from build123d import *

# Parameters (mm, degrees)
SKETCH1_R               = 55
SKETCH1_W               = 30.631456328
SKETCH1_H               = 90
HOUSING_DEPTH           = 30
INTERNALCUT_DEPTH       = 27
SKETCH7_W               = 72
SKETCH7_H               = 25
DISPLAYCUT_DEPTH        = 27
SKETCH11_R              = 18
WICHARGERCUT_DEPTH      = 1
SKETCH14_W              = 4.6
SKETCH14_H              = 6.1
BTNINTERNALCUT_DEPTH    = 1
SKETCH16_R              = 1.5
BTNEXTERNALCUT_DEPTH    = 116.280995765
SKETCH18_R              = 6
BUZZEREXTERNALCUT_DEPTH = 1
SKETCH20_R              = 0.35
BUZZERINTERNALCUT_DEPTH = 116.863890151
SKETCH23_W              = 3.7
SKETCH23_H              = 8.5
SWITCHINTERNALCUT_DEPTH = 1
SKETCH25_W              = 1.7
SKETCH25_H              = 3.6
SWITCHEXTERNALCUT_DEPTH = 124.821406818
MICROUSBCUT_DEPTH       = 128.13897565
SKETCH29_R              = 3.5
SKETCH29_R_2            = 1.5
BOSS_EXTRUDE1_DEPTH     = 27
SKETCH30_R              = 1.5
CUT_EXTRUDE1_DEPTH      = 83.757833161
CUT_EXTRUDE1_DEPTH_BACK = 83.757833161
SKETCH31_W              = 59.5
SKETCH31_H              = 2
BOSS_EXTRUDE3_DEPTH     = 5


with BuildPart() as part:
    # Sketch1 → Housing (new body)
    with BuildSketch(Plane(origin=(0, 0, 0), x_dir=(1, 0, 0), z_dir=(0, 1, 0))):
        Circle(SKETCH1_R)
        with Locations((40.315728164, -0.0001724)):
            Rectangle(SKETCH1_W, SKETCH1_H)
    extrude(amount=HOUSING_DEPTH)

    # Sketch8 → InternalCut (cut)
    with BuildSketch(Plane(origin=(0, 30, 0), x_dir=(1, 0, 0), z_dir=(0, 1, 0))):
        with BuildLine():
            ThreePointArc((29.731697916, 40.1998276), (-49.999999999, 0.000289929), (29.73123171, -40.2001724))
            Line((29.73123171, -40.2001724), (19.336952431, -40.2001724))
            Line((19.336952431, -40.2001724), (19.336952431, 40.1998276))
            Line((19.336952431, 40.1998276), (29.731697916, 40.1998276))
        make_face()
        with BuildLine():
            Line((19.336952431, -40.2001724), (29.73123171, -40.2001724))
            ThreePointArc((29.73123171, -40.2001724), (44.646173327, -22.510424413), (50, 0))
            ThreePointArc((50, 0), (44.646303855, 22.510165528), (29.731697916, 40.1998276))
            Line((29.731697916, 40.1998276), (19.336952431, 40.1998276))
            Line((19.336952431, 40.1998276), (19.336952431, -40.2001724))
        make_face()
        with BuildLine():
            Line((29.73123171, -40.2001724), (50.631456328, -40.2001724))
            Line((50.631456328, -40.2001724), (50.631456328, 40.1998276))
            Line((50.631456328, 40.1998276), (29.731697916, 40.1998276))
            ThreePointArc((29.731697916, 40.1998276), (44.646303855, 22.510165528), (50, 0))
            ThreePointArc((50, 0), (44.646173327, -22.510424413), (29.73123171, -40.2001724))
        make_face()
    extrude(amount=-INTERNALCUT_DEPTH, mode=Mode.SUBTRACT)

    # Sketch7 → DisplayCut (cut)
    with BuildSketch(Plane(origin=(55.631456328, 0, 0), x_dir=(0, 0, -1), z_dir=(1, 0, 0))):
        with Locations((-0.0001724, 22.5)):
            Rectangle(SKETCH7_W, SKETCH7_H)
    extrude(amount=-DISPLAYCUT_DEPTH, mode=Mode.SUBTRACT)

    # Sketch11 → WiChargerCut (cut)
    with BuildSketch(Plane(origin=(0, 3, 0), x_dir=(1, 0, 0), z_dir=(0, 1, 0))):
        with Locations(Location((0, 0, 0), (0, 0, 270))):
            Circle(SKETCH11_R)
    extrude(amount=-WICHARGERCUT_DEPTH, mode=Mode.SUBTRACT)

    # Sketch14 → BtnInternalCut (cut)
    with BuildSketch(Plane(origin=(4.856972308, 3, -39.46084295), x_dir=(1, 0, 0), z_dir=(0, 1, 0))):
        with Locations((-0.204569722, -74.22253241)):
            Rectangle(SKETCH14_W, SKETCH14_H)
    extrude(amount=-BTNINTERNALCUT_DEPTH, mode=Mode.SUBTRACT)

    # Sketch16 → BtnExternalCut (cut, through all)
    with BuildSketch(Plane(origin=(4.856972308, 2, -39.46084295), x_dir=(1, 0, 0), z_dir=(0, 1, 0))):
        with Locations(Location((-0.204569722, -74.22253241, 0), (0, 0, 270))):
            Circle(SKETCH16_R)
    extrude(amount=-BTNEXTERNALCUT_DEPTH, mode=Mode.SUBTRACT)

    # Sketch18 → BuzzerExternalCut (cut)
    with BuildSketch(Plane(origin=(12.790381818, 3, 34.693395374), x_dir=(1, 0, 0), z_dir=(0, 1, 0))):
        with Locations(Location((-25.006618322, 0, 0), (0, 0, 270))):
            Circle(SKETCH18_R)
    extrude(amount=-BUZZEREXTERNALCUT_DEPTH, mode=Mode.SUBTRACT)

    # Sketch20 → BuzzerInternalCut (cut, through all)
    with BuildSketch(Plane(origin=(12.790381818, 2, 34.693395374), x_dir=(1, 0, 0), z_dir=(0, 1, 0))):
        with Locations(Location((-24.042348329, 4.522315504, 0), (0, 0, 270))):
            Circle(SKETCH20_R)
        with Locations(Location((-26.042348329, 3.020429056, 0), (0, 0, 270))):
            Circle(SKETCH20_R)
        with Locations(Location((-28.042348329, 3.020429056, 0), (0, 0, 270))):
            Circle(SKETCH20_R)
        with Locations(Location((-30.042348329, 1.518542609, 0), (0, 0, 270))):
            Circle(SKETCH20_R)
        with Locations(Location((-30.042348329, 0.016656161, 0), (0, 0, 270))):
            Circle(SKETCH20_R)
        with Locations(Location((-30.042348329, -1.485230286, 0), (0, 0, 270))):
            Circle(SKETCH20_R)
        with Locations(Location((-28.042348329, 0.016656161, 0), (0, 0, 270))):
            Circle(SKETCH20_R)
        with Locations(Location((-28.042348329, 1.518542609, 0), (0, 0, 270))):
            Circle(SKETCH20_R)
        with Locations(Location((-28.042348329, -1.485230286, 0), (0, 0, 270))):
            Circle(SKETCH20_R)
        with Locations(Location((-28.042348329, -2.987116733, 0), (0, 0, 270))):
            Circle(SKETCH20_R)
        with Locations(Location((-26.042348329, 0.016656161, 0), (0, 0, 270))):
            Circle(SKETCH20_R)
        with Locations(Location((-26.042348329, 1.518542609, 0), (0, 0, 270))):
            Circle(SKETCH20_R)
        with Locations(Location((-26.042348329, -1.485230286, 0), (0, 0, 270))):
            Circle(SKETCH20_R)
        with Locations(Location((-26.042348329, -2.987116733, 0), (0, 0, 270))):
            Circle(SKETCH20_R)
        with Locations(Location((-26.042348329, -4.489003181, 0), (0, 0, 270))):
            Circle(SKETCH20_R)
        with Locations(Location((-24.042348329, -4.489003181, 0), (0, 0, 270))):
            Circle(SKETCH20_R)
        with Locations(Location((-24.042348329, -2.987116733, 0), (0, 0, 270))):
            Circle(SKETCH20_R)
        with Locations(Location((-24.042348329, -1.485230286, 0), (0, 0, 270))):
            Circle(SKETCH20_R)
        with Locations(Location((-24.042348329, 0.016656161, 0), (0, 0, 270))):
            Circle(SKETCH20_R)
        with Locations(Location((-24.042348329, 1.518542609, 0), (0, 0, 270))):
            Circle(SKETCH20_R)
        with Locations(Location((-24.042348329, 3.020429056, 0), (0, 0, 270))):
            Circle(SKETCH20_R)
        with Locations(Location((-22.042348329, 3.020429056, 0), (0, 0, 270))):
            Circle(SKETCH20_R)
        with Locations(Location((-22.042348329, 1.518542609, 0), (0, 0, 270))):
            Circle(SKETCH20_R)
        with Locations(Location((-22.042348329, 0.016656161, 0), (0, 0, 270))):
            Circle(SKETCH20_R)
        with Locations(Location((-22.042348329, -1.485230286, 0), (0, 0, 270))):
            Circle(SKETCH20_R)
        with Locations(Location((-22.042348329, -2.987116733, 0), (0, 0, 270))):
            Circle(SKETCH20_R)
        with Locations(Location((-20.042348329, -1.485230286, 0), (0, 0, 270))):
            Circle(SKETCH20_R)
        with Locations(Location((-20.042348329, 0.016656161, 0), (0, 0, 270))):
            Circle(SKETCH20_R)
        with Locations(Location((-20.042348329, 1.518542609, 0), (0, 0, 270))):
            Circle(SKETCH20_R)
        with Locations(Location((-26.042348329, 4.522315504, 0), (0, 0, 270))):
            Circle(SKETCH20_R)
    extrude(amount=-BUZZERINTERNALCUT_DEPTH, mode=Mode.SUBTRACT)

    # Sketch23 → SwitchInternalCut (cut)
    with BuildSketch(Plane(origin=(-6.532000561, 3, 48.360753742), x_dir=(1, 0, 0), z_dir=(0, 1, 0))):
        with Locations((23.409044431, 13.599064282)):
            Rectangle(SKETCH23_W, SKETCH23_H)
    extrude(amount=-SWITCHINTERNALCUT_DEPTH, mode=Mode.SUBTRACT)

    # Sketch25 → SwitchExternalCut (cut, through all)
    with BuildSketch(Plane(origin=(-6.532000561, 2, 48.360753742), x_dir=(1, 0, 0), z_dir=(0, 1, 0))):
        with Locations((23.409044431, 13.599064282)):
            Rectangle(SKETCH25_W, SKETCH25_H)
    extrude(amount=-SWITCHEXTERNALCUT_DEPTH, mode=Mode.SUBTRACT)

    # Sketch28 → MicroUSBCut (cut, through all)
    with BuildSketch(Plane(origin=(55.631456328, 0, 0), x_dir=(0, 0, -1), z_dir=(1, 0, 0))):
        with BuildLine():
            Line((-3.7251724, 13.5), (3.7248276, 13.5))
            ThreePointArc((3.7248276, 13.5), (5.4748276, 11.75), (3.7248276, 10))
            Line((3.7248276, 10), (-3.7251724, 10))
            ThreePointArc((-3.7251724, 10), (-5.4751724, 11.75), (-3.7251724, 13.5))
        make_face()
    extrude(amount=-MICROUSBCUT_DEPTH, mode=Mode.SUBTRACT)

    # Sketch29 → Boss-Extrude1 (add)
    with BuildSketch(Plane(origin=(0, 3, 0), x_dir=(1, 0, 0), z_dir=(0, 1, 0))):
        with Locations((-24.932520247, 43.184391828)):
            Circle(SKETCH29_R)
        with Locations((-24.932520247, 43.184391828)):
            Circle(SKETCH29_R_2, mode=Mode.SUBTRACT)
        with Locations((-25, -43.301270189)):
            Circle(SKETCH29_R)
        with Locations((-25, -43.301270189)):
            Circle(SKETCH29_R_2, mode=Mode.SUBTRACT)
        with Locations((29.731697916, 40.1998276)):
            Circle(SKETCH29_R)
        with Locations((29.731697916, 40.1998276)):
            Circle(SKETCH29_R_2, mode=Mode.SUBTRACT)
        with Locations((29.73123171, -40.2001724)):
            Circle(SKETCH29_R)
        with Locations((29.73123171, -40.2001724)):
            Circle(SKETCH29_R_2, mode=Mode.SUBTRACT)
    extrude(amount=BOSS_EXTRUDE1_DEPTH)

    # Sketch30 → Cut-Extrude1 (cut, two sides)
    with BuildSketch(Plane(origin=(0, 3, 0), x_dir=(1, 0, 0), z_dir=(0, 1, 0))) as cut_extrude1_sk:
        with Locations(Location((29.731697916, 40.1998276, 0), (0, 0, 270))):
            Circle(SKETCH30_R)
        with Locations(Location((-25, -43.301270189, 0), (0, 0, 270))):
            Circle(SKETCH30_R)
        with Locations(Location((29.73123171, -40.2001724, 0), (0, 0, 270))):
            Circle(SKETCH30_R)
        with Locations(Location((-25, 43.301270189, 0), (0, 0, 270))):
            Circle(SKETCH30_R)
    extrude(amount=CUT_EXTRUDE1_DEPTH, mode=Mode.SUBTRACT)
    extrude(cut_extrude1_sk.sketch, amount=-CUT_EXTRUDE1_DEPTH_BACK, mode=Mode.SUBTRACT)

    # Sketch31 → Boss-Extrude3 (add)
    with BuildSketch(Plane(origin=(0, 3, 0), x_dir=(1, 0, 0), z_dir=(0, 1, 0))):
        with BuildLine():
            Line((-26.280928, 39.954562648), (-30.060487747, 39.954562648))
            ThreePointArc((-30.060487747, 39.954562648), (-32.181707413, 38.266665755), (-34.208331283, 36.466286771))
            Line((-34.208331283, 36.466286771), (-34.208331283, 33.954562648))
            Line((-34.208331283, 33.954562648), (28.791668717, 33.954562648))
            Line((28.791668717, 33.954562648), (28.791668717, 36.82842654))
            ThreePointArc((28.791668717, 36.82842654), (27.020136784, 37.98681241), (26.240302048, 39.954562648))
            Line((26.240302048, 39.954562648), (-23.584112493, 39.954562648))
            ThreePointArc((-23.584112493, 39.954562648), (-24.932520247, 39.684391828), (-26.280928, 39.954562648))
        make_face()
        with Locations((-2.708331283, 36.954562648)):
            Rectangle(SKETCH31_W, SKETCH31_H, mode=Mode.SUBTRACT)
    extrude(amount=BOSS_EXTRUDE3_DEPTH)


solid = part.part
Could you check a few things on this model? Use its own coordinates, in mm. A direction names the side the tool comes from. Round coordinates to 2 decimals unless told otherwise and drop trailing zeros. Write each loop counter-clockwise with the first axis right and the second up, starting at its lowest first coordinate (ties: lowest second). Pieces come first, ordered by that corner, then holes. Notation, with made-up numbers: (60, 37.5) -> (81, 37.5) arc R27 ccw to (81, 57.5) -> close; hole circle Ø5 at (13, 19.5). An arc over 180 degrees is marked (long way). Use a Markdown table: item, result.
1. Which directions (+Z, -Z, +X, -X, +Y, -Y) give clear straight access to the entire face, cutting with the end or side of a thin tool? Please do faces 3 (the face through (55.631, 8, 1)), 4 (the face through (53, 20, 36)), 5 (the face through (15.6, 2, 34.7)), 6 (the face through (-52, 13.5, 0)).
Answer key:
| item | result |
|---|---|
| face 3 | +Z, -Z, +X, +Y, -Y |
| face 4 | +X, +Y |
| face 5 | +Y |
| face 6 | +X, -X |
2. If we section it at D-D (y = 24): List the corners of the cut face in (x, z) for me.
Answer key:
| item | result |
|---|---|
| outline | (-27.97, -41.45) arc R50 cw to (-27.97, 41.45) arc R3.5 ccw to (-21.91, 44.94) arc R50 cw to (26.85, 42.18) arc R3.5 ccw (long way) to (33.23, 40.2) -> (50.63, 40.2) -> (50.63, 36) -> (55.63, 36) -> (55.63, 45) -> (31.62, 45) arc R55 ccw (long way) to (31.62, -45) -> (55.63, -45) -> (55.63, -36) -> (50.63, -36) -> (50.63, -40.2) -> (33.23, -40.2) arc R3.5 ccw (long way) to (26.85, -42.18) arc R50 cw to (-21.91, -44.95) arc R3.5 ccw (long way) to start; hole circle Ø3 at (-25, 43.3); hole (-26.26, -42.49) arc R1.5 ccw (long way) to (-23.67, -43.99) arc R1.5 ccw (long way) to start; hole circle Ø3 at (29.73, -40.2); hole circle Ø3 at (29.73, 40.2) |
3. Please list where these lines run through material, in increasing order: probe 1 along X at (y, z) = (16, 39); probe 2 along X at (y, z) = (7, 37.5); probe 3 along Y at (x, z) = (-12, -31.5).
Answer key:
| item | result |
|---|---|
| probe 1 | x = -38.78 to -31.29, 26.44 to 28.83, 30.63 to 33.02, 50.63 to 55.63 |
| probe 2 | x = -40.23 to -33.07, 27.5 to 31.96, 50.63 to 55.63 |
| probe 3 | y = 0 to 3 |
4. We'd pull the mould along Z, two halves only. Please class faces 1 (the face through (-25, 30, 40)), 2 (the face through (-3, 5, -35.955)): +Z half, -Z half, draft (parallel to the pull), parting line (faces both ways), or undercut.
Answer key:
| item | result |
|---|---|
| face 1 | draft |
| face 2 | undercut |
5. For pin 1 Ø3 at (x, y) = (-28.5, 5.5) entering from -Z; pin 2 Ø2 at (x, y) = (19, 24) entering from -Z; pin 3 Ø2 at (x, y) = (-30.5, 26) entering from -Z; pin 4 Ø5.5 at (x, z) = (-52, -0.5) entering from -Y, each with a flat end and sliding along its axis, tell me the tip position at first contact or that it passes through.
Answer key:
| item | result |
|---|---|
| pin 1 | stops at z = -47.92 |
| pin 2 | stops at z = -51.97 |
| pin 3 | stops at z = -46.42 |
| pin 4 | stops at y = 0 |
6. If we section it at B-B (y = 11.75): List the corners of the cut face in (x, z) for me.
Answer key:
| item | result |
|---|---|
| outline | (-54.73, -5.47) arc R55 ccw to (31.62, -45) -> (55.63, -45) -> (55.63, -36) -> (50.63, -36) -> (50.63, -40.2) -> (33.23, -40.2) arc R3.5 ccw (long way) to (26.85, -42.18) arc R50 cw to (-21.91, -44.95) arc R3.5 ccw (long way) to (-27.97, -41.45) arc R50 cw to (-49.7, -5.47) -> close; (-54.73, 5.48) -> (-49.7, 5.48) arc R50 cw to (-27.97, 41.45) arc R3.5 ccw to (-21.91, 44.94) arc R50 cw to (26.85, 42.18) arc R3.5 ccw (long way) to (33.23, 40.2) -> (50.63, 40.2) -> (50.63, 36) -> (55.63, 36) -> (55.63, 45) -> (31.62, 45) arc R55 ccw to start; hole circle Ø3 at (-25, 43.3); hole (-26.26, -42.49) arc R1.5 ccw (long way) to (-23.67, -43.99) arc R1.5 ccw (long way) to start; hole circle Ø3 at (29.73, -40.2); hole circle Ø3 at (29.73, 40.2) |
7. If we section it at A-A (z = 0): List the corners of the cut face in (x, y) for me.
Answer key:
| item | result |
|---|---|
| outline | (-55, 0) -> (55.63, 0) -> (55.63, 10) -> (50.63, 10) -> (50.63, 3) -> (18, 3) -> (18, 2) -> (-18, 2) -> (-18, 3) -> (-50, 3) -> (-50, 10) -> (-55, 10) -> close; (-55, 13.5) -> (-50, 13.5) -> (-50, 30) -> (-55, 30) -> close |
8. If we section it at C-C (x = 0): List the corners of the cut face in (y, z) for me.
Answer key:
| item | result |
|---|---|
| outline | (0, -55) -> (30, -55) -> (30, -50) -> (3, -50) -> (3, -39.95) -> (8, -39.95) -> (8, -37.95) -> (3, -37.95) -> (3, -35.95) -> (8, -35.95) -> (8, -33.95) -> (3, -33.95) -> (3, -18) -> (2, -18) -> (2, 18) -> (3, 18) -> (3, 50) -> (30, 50) -> (30, 55) -> (0, 55) -> close |
